Verification items for the finished model (mm, model axes). A direction names the side the tool comes from. Give positions to 0.01 mm unless a question says otherwise; leave off trailing zeros. Write each loop counter-clockwise with the first axis right and the second up, starting at its lowest first coordinate (ties: lowest second). Pieces come first, ordered by that corner, then holes. Notation, with made-up numbers: (2.5, -18.5) - (41.5, -18.5) arc R12 cw to (41.5, -5.5) - close; hole circle Ø2 at (66, -22). An arc over 180 degrees is marked (long way). Answer as a JSON object with one key per item and string values. Group by question number.
Item 1: Sectioned sample at A-A, the plane y = -0.25. Record the boundary of the cut face in (x, z).
Item 2: Scan lines: line 1 along X through (y, z) = (2.5, 5); line 2 along X through (y, z) = (4.25, 8.5); line 3 along Y through (x, z) = (-16, 11). Record each from-to range of solid material in increasing order. Write a range as [from, to].
Item 3: Draft check along X on faces 6 (the face through (-27, -1, 6)), 7 (the face through (-22.513, -3.591, 5.195)), 8 (the face through (0, 10, 11)). Enter one of: +X half, -X half, draft (parallel to the pull), parting line (faces both ways), or undercut.
Item 4: Sectioned sample at B-B, the plane z = 5. Record the boundary of the cut face in (x, y).
Item 5: Sectioned sample at D-D, the plane x = -12.5. Record the boundary of the cut face in (y, z).
Item 6: Sectioned sample at C-C, the plane x = -24. Record the boundary of the cut face in (y, z).
Item 7: Tool access check on faces 1 (the face through (0, 8, 10)), 2 (the face through (14.8, 7.1, 11.5)), 3 (the face through (25.487, -3.591, 5.195)), 4 (the face through (21, 0, 7)), 5 (the face through (0, 6, 12)). Record the directions out of +Z, -Z, +X, -X, +Y, -Y that give a thin tool (end or side, any length) a straight path to the whole face; none if there is none.
Item 8: Go/stop test with flat-tipped pins: pin 1 (2 mm diameter, centred on x = 9.5, y = 5.5, fed in from -Z); pin 2 (2.5 mm diameter, centred on x = 5.5, z = 11.5, fed in from -Y); pin 3 (1.8 mm diameter, centred on x = -24, z = 5, fed in from -Y). Record where each tip stops, or that it passes through.
```python
from build123d import *

# Parameters (mm, degrees)
SKETCH_1_W          = 54
SKETCH_1_H          = 20
EXTRUDE_1_DEPTH     = 13
SKETCH_2_W          = 42
SKETCH_2_H          = 16
CUT_EXTRUDE_1_DEPTH = 32.591137998
SKETCH_3_R          = 1.5
CUT_EXTRUDE_2_DEPTH = 32.591137998
SKETCH_4_R          = 1.5
CUT_EXTRUDE_3_DEPTH = 13
SKETCH_5_W          = 42
SKETCH_5_H          = 10
CUT_EXTRUDE_4_DEPTH = 37.027767069
CHAMFER_1_SIZE      = 2
CHAMFER_2_SIZE      = 2
CHAMFER_3_SIZE      = 0.4


with BuildPart() as part:
    # 草圖1 → 填料-伸長1 (new body)
    with BuildSketch(Plane.XY):
        Rectangle(SKETCH_1_W, SKETCH_1_H)
    extrude(amount=EXTRUDE_1_DEPTH)

    # 草圖2 → 除料-伸長1 (cut, through all)
    with BuildSketch(Plane.XY.offset(13)):
        with Locations((0, -2)):
            Rectangle(SKETCH_2_W, SKETCH_2_H)
    extrude(amount=-CUT_EXTRUDE_1_DEPTH, mode=Mode.SUBTRACT)

    # 草圖3 → 除料-伸長2 (cut, through all)
    with BuildSketch(Plane.XY.offset(13)):
        with Locations((-16, 8)):
            Circle(SKETCH_3_R)
        with Locations((16, 8)):
            Circle(SKETCH_3_R)
    extrude(amount=-CUT_EXTRUDE_2_DEPTH, mode=Mode.SUBTRACT)

    # 草圖4 → 除料-伸長3 (cut)
    with BuildSketch(Plane.XZ.offset(10)):
        with Locations(Location((-24, 5, 0), (0, 0, 270))):
            Circle(SKETCH_4_R)
        with Locations(Location((24, 5, 0), (0, 0, 270))):
            Circle(SKETCH_4_R)
    extrude(amount=-CUT_EXTRUDE_3_DEPTH, mode=Mode.SUBTRACT)

    # 草圖5 → 除料-伸長4 (cut, through all)
    with BuildSketch(Plane(origin=(0, 10, 0), x_dir=(1, 0, 0), z_dir=(0, 1, 0))):
        with Locations((0, -5)):
            Rectangle(SKETCH_5_W, SKETCH_5_H)
    extrude(amount=-CUT_EXTRUDE_4_DEPTH, mode=Mode.SUBTRACT)

    # 導角1
    chamfer_1_edges = [part.edges().sort_by_distance(p)[0] for p in [
        (-27, 10, 6.5),
        (27, 10, 6.5),
    ]]
    chamfer(chamfer_1_edges, length=CHAMFER_1_SIZE)

    # 導角2
    chamfer_2_edges = [part.edges().sort_by_distance(p)[0] for p in [
        (21, 6, 11.5),
        (-21, 6, 11.5),
    ]]
    chamfer(chamfer_2_edges, length=CHAMFER_2_SIZE)

    # 導角3
    chamfer_3_edges = [part.edges().sort_by_distance(p)[0] for p in [
        (-21, 7, 10),
        (21, 7, 10),
    ]]
    chamfer(chamfer_3_edges, length=CHAMFER_3_SIZE)


solid = part.part
```
Geometry check:
{
 "1": {"outline": "(-27, 0) - (-21, 0) - (-21, 13) - (-27, 13) - close; (21, 0) - (27, 0) - (27, 13) - (21, 13) - close; hole circle Ø3 at (-24, 5); hole circle Ø3 at (24, 5)"},
 "2": {"line 1": "[-27, -25.5], [-22.5, -21], [21, 22.5], [25.5, 27]", "line 2": "[-27, -21], [21, 27]", "line 3": "[6, 6.5], [9.5, 10]"},
 "3": {"face 6": "-X half", "face 7": "undercut", "face 8": "draft"},
 "4": {"outline": "(-27, -10) - (-25.5, -10) - (-25.5, 3) - (-22.5, 3) - (-22.5, -10) - (-21, -10) - (-21, 10) - (-25, 10) - (-27, 8) - close; (21, -10) - (22.5, -10) - (22.5, 3) - (25.5, 3) - (25.5, -10) - (27, -10) - (27, 8) - (25, 10) - (21, 10) - close"},
 "5": {"outline": "(6, 10) - (10, 10) - (10, 13) - (6, 13) - close"},
 "6": {"outline": "(-10, 0) - (10, 0) - (10, 13) - (-10, 13) - (-10, 6.5) - (3, 6.5) - (3, 3.5) - (-10, 3.5) - close"},
 "7": {"face 1": "-Z, +Y, -Y", "face 2": "+Z, -Z", "face 3": "-Y", "face 4": "-Z, -Y", "face 5": "+Z, -Z, -Y"},
 "8": {"pin 1": "z = 10", "pin 2": "y = 6", "pin 3": "y = 3"}
}
